Input: part model. Units: mm. Frame: model coordinates. A direction names the side the tool comes from. Round coordinates to 2 decimals unless told otherwise and drop trailing zeros. One line per item, written item: value. Start each with the question number.
from build123d import *

# Parameters (mm, degrees)
SHELL1_T  = -3.0734
FILLET1_R = 5.08


with BuildPart() as part:
    # Sketch1 → Loft1 section 0
    with BuildSketch(Plane.XY):
        with BuildLine():
            Line((20.1168, 12.5095), (-20.1168, 12.5095))
            Line((-20.1168, 12.5095), (-20.1168, -12.5095))
            Line((-20.1168, -12.5095), (20.1168, -12.5095))
            Line((20.1168, -12.5095), (20.1168, 12.5095))
        make_face()
    # 3DSketch1 → Loft1 section 1
    with BuildSketch(Plane(origin=(-20.1168, -11.811, 130.175), x_dir=(0.9998754744294865, 0.015780862917132092, 0), z_dir=(0, 0, 1))):
        with BuildLine():
            Line((0, 0), (40.228589888, -0.634920926))
            Line((40.228589888, -0.634920926), (40.238610736, 0))
            Line((40.238610736, 0), (0.010020848, 0.634920926))
            Line((0.010020848, 0.634920926), (0, 0))
        make_face()
    loft()

    # Shell1
    shell1_openings = [part.faces().sort_by_distance(p)[0] for p in [
        (0, 0, 0),
    ]]
    offset(amount=SHELL1_T, openings=shell1_openings, kind=Kind.INTERSECTION)

    # Fillet1
    # the kernel refuses this fillet: 5.08 mm, written as the material it takes off along each edge
    with BuildSketch(Plane(origin=(20.1168, 14.78295414, -12.494855192), x_dir=(-1, 0, 0), z_dir=(0, -0.1790121369959656, 0.9838468655274243))) as fillet1_piece_1:
        with BuildLine():
            CenterArc((FILLET1_R, FILLET1_R), FILLET1_R, 180, 90)
            Line((0, FILLET1_R), (0, 0))
            Line((0, 0), (FILLET1_R, 0))
        make_face()
    extrude(amount=157.712257691, mode=Mode.SUBTRACT)
    with BuildSketch(Plane(origin=(-20.1168, 14.78295414, -12.494855192), x_dir=(1, 0, 0), z_dir=(0, -0.17901213699596547, 0.9838468655274243))) as fillet1_piece_2:
        with BuildLine():
            CenterArc((FILLET1_R, -FILLET1_R), FILLET1_R, 90, 90)
            Line((0, -FILLET1_R), (0, 0))
            Line((0, 0), (FILLET1_R, 0))
        make_face()
    extrude(amount=157.712257691, mode=Mode.SUBTRACT)
    with BuildSketch(Plane(origin=(-20.1168, -12.57764536, -12.699817172), x_dir=(0, 0.9999856041181256, -0.005365776412341061), z_dir=(0, 0.0053657764123410615, 0.9999856041181258)), Plane(origin=(20.1168, -12.57764536, -12.699817172), x_dir=(-1, 0, 0), z_dir=(0, 0.0053657764123410485, 0.9999856041181258))) as fillet1_piece_3:
        with BuildLine():
            CenterArc((FILLET1_R, -FILLET1_R), FILLET1_R, 90, 90)
            Line((0, -FILLET1_R), (0, 0))
            Line((0, 0), (FILLET1_R, 0))
        make_face()
    extrude(amount=155.576874011, mode=Mode.SUBTRACT)


solid = part.part
1. Set-up query: faces 1 (the face through (-18.668, -10.638, 64.169)), 2 (the face through (18.67, -0.68, 63.93)), 3 (the face through (17.043, -4, 39)). Return all of +Z, -Z, +X, -X, +Y, -Y with unobstructed straight access to the full face (end or side cutting, diameter ignored); none if empty.
2. Line query: line 1 (X direction, y = -0.5, z = 26); line 2 (Y direction, x = 2, z = 87); line 3 (Y direction, x = -0.5, z = 30.5). Output: solid intervals per line, ascending. Write a range as from..to.
3. Pull-direction query (Y, two-part tool) for faces 4 (the face through (-18.6, -0.6, 63.9)), 5 (the face through (-17.043, -3, 39)), 6 (the face through (18.589, -10.717, 64.169)); classes: released by +Y, released by -Y, zero draft, split by the parting line, or undercut.
4. Pin query (flat end, axial travel): pin 1 (5 mm diameter, centred on x = -3.5, z = 13.5, fed in from +Y); pin 2 (4 mm diameter, centred on y = -6.5, z = 109.5, fed in from +X); pin 3 (10 mm diameter, centred on x = 8, z = 70, fed in from -Y); pin 4 (8 mm diameter, centred on y = 2.5, z = 46, fed in from +X). Return the tip coordinate at first contact, or that it passes through.
Solved:
1. face 1: +Z, -X, -Y
1. face 2: +Z, +X, +Y
1. face 3: -Z
2. line 1: x = -20.12..-17.04, 17.04..20.12
2. line 2: y = -12.04..-8.97, -6.44..-3.32
2. line 3: y = -12.35..-9.27, 3.84..6.96
3. face 4: released by +Y
3. face 5: undercut
3. face 6: released by -Y
4. pin 1: stops at y = 10.51
4. pin 2: stops at x = 18.19
4. pin 3: stops at y = -12.16
4. pin 4: stops at x = 20.12
